```python
from build123d import *

# Parameters (mm, degrees)
SALIENTE_EXTRUIR2_DEPTH = 10
ESCALA1_SCALE           = 0.5


with BuildPart() as part:
    # Croquis1 → Saliente-Extruir2 (new body)
    with BuildSketch(Plane(origin=(0, 0, 0), x_dir=(1, 0, 0), z_dir=(0, 1, 0))):
        with BuildLine():
            Line((347.768463119, -7.519240019), (347.768463119, 12.480759981))
            Line((347.768463119, 12.480759981), (-82.231536881, 17.480759981))
            Line((-82.231536881, 17.480759981), (-89.231536881, 17.480759981))
            ThreePointArc((-89.231536881, 17.480759981), (-89.938643662, 17.187866762), (-90.231536881, 16.480759981))
            Line((-90.231536881, 16.480759981), (-90.231536881, 13.480759981))
            ThreePointArc((-90.231536881, 13.480759981), (-89.938643662, 12.7736532), (-89.231536881, 12.480759981))
            Line((-89.231536881, 12.480759981), (-82.231536881, 12.480759981))
            Line((-82.231536881, 12.480759981), (-82.231536881, -7.519240019))
            Line((-82.231536881, -7.519240019), (-89.231536881, -7.519240019))
            ThreePointArc((-89.231536881, -7.519240019), (-89.938643662, -7.812133238), (-90.231536881, -8.519240019))
            Line((-90.231536881, -8.519240019), (-90.231536881, -11.519240019))
            ThreePointArc((-90.231536881, -11.519240019), (-89.938643662, -12.2263468), (-89.231536881, -12.519240019))
            Line((-89.231536881, -12.519240019), (-82.231536881, -12.519240019))
            Line((-82.231536881, -12.519240019), (347.768463119, -7.519240019))
        make_face()
        Polygon((-35.970310827, -6.981318786), (-35.970310827, 11.942838748), (-59.970310827, 12.221908515), (-59.970310827, -7.260388554), align=None, mode=Mode.SUBTRACT)
        Polygon((-6.36676246, -6.637091479), (-6.36676246, 11.598611441), (-30.970310827, 11.884699213), (-30.970310827, -6.923179251), align=None, mode=Mode.SUBTRACT)
        Polygon((24.032508683, -6.283611582), (24.032508683, 11.245131544), (-1.36676246, 11.540471906), (-1.36676246, -6.578951945), align=None, mode=Mode.SUBTRACT)
        Polygon((54.471653082, -5.929668043), (54.471653082, 10.891188004), (29.032508683, 11.186992009), (29.032508683, -6.225472048), align=None, mode=Mode.SUBTRACT)
        Polygon((83.209124846, -5.595511395), (83.209124846, 10.557031356), (59.471653082, 10.83304847), (59.471653082, -5.871528508), align=None, mode=Mode.SUBTRACT)
        Polygon((112.395607474, -5.25613369), (112.395607474, 10.217653651), (88.209124846, 10.498891821), (88.209124846, -5.53737186), align=None, mode=Mode.SUBTRACT)
        Polygon((142.246515855, -4.909030104), (142.246515855, 9.870550065), (117.395607474, 10.159514116), (117.395607474, -5.197994155), align=None, mode=Mode.SUBTRACT)
        Polygon((171.437834583, -4.569596165), (171.437834583, 9.531116127), (147.246515855, 9.81241053), (147.246515855, -4.850890569), align=None, mode=Mode.SUBTRACT)
        Polygon((200.288401316, -4.234124459), (200.288401316, 9.19564442), (176.437834583, 9.472976592), (176.437834583, -4.51145663), align=None, mode=Mode.SUBTRACT)
        Polygon((229.28834427, -3.89691582), (229.28834427, 8.858435781), (205.288401316, 9.137504885), (205.288401316, -4.175984924), align=None, mode=Mode.SUBTRACT)
        Polygon((258.357613703, -3.558901059), (258.357613703, 8.52042102), (234.28834427, 8.800296246), (234.28834427, -3.838776285), align=None, mode=Mode.SUBTRACT)
        Polygon((287.325919365, -3.222060295), (287.325919365, 8.183580257), (263.357613703, 8.462281486), (263.357613703, -3.500761524), align=None, mode=Mode.SUBTRACT)
        Polygon((315.709556101, -2.892018008), (315.709556101, 7.853537969), (292.325919365, 8.125440722), (292.325919365, -3.163920761), align=None, mode=Mode.SUBTRACT)
        Polygon((342.768463119, -2.577379554), (342.768463119, 7.538899516), (320.709556101, 7.795398434), (320.709556101, -2.833878473), align=None, mode=Mode.SUBTRACT)
        Polygon((-64.970310827, -7.318528088), (-64.970310827, 12.28004805), (-72.387230354, 12.3662913), (-79.231536881, 6.910670608), (-79.231536881, -1.949150646), (-72.387230358, -7.404771339), align=None, mode=Mode.SUBTRACT)
    extrude(amount=SALIENTE_EXTRUIR2_DEPTH)


with BuildPart() as part_1:
    # Escala1: scaled about (123.080377325, 5, -2.480759981)
    add(part.part.scale(ESCALA1_SCALE).moved(Location((61.540188663, 2.5, -1.24037999))))


solid = part_1.part
```
Here's how the part is built. I have some questions about the finished solid (model axes, mm). Coordinates: 2 decimals unless noted, no trailing zeros. Order: outer loops, then holes, each group sorted by start corner. A loop starts at its lowest first (then second) coordinate and runs counter-clockwise, first axis right, second up.
1) Imagine slicing it at A-A on x = 36.5. List the corners of the cut face in (y, z) for me.
2) Will this pin go through, and if not, where does the flat tip stop? pin 1 (2.5 mm diameter, centred on y = 5, z = -0.5, fed in from -X).
3) I need wall thicknesses on line 1 (Z direction, x = 34, y = 7.15); line 2 (Z direction, x = 171, y = 6.45); line 3 (Z direction, x = 192, y = 2.85). Which ranges of each line are inside material? Lowest first, please.
4) Imagine slicing it at B-B on y = 4.6. State how many separate pieces and enclosed holes the cut face has, and give its area (3 significant figures).
Response values:
1. outline: (2.5, -9.79) - (7.5, -9.79) - (7.5, -7.29) - (2.5, -7.29) - close; (2.5, 2.33) - (7.5, 2.33) - (7.5, 4.83) - (2.5, 4.83) - close
2. pin 1: stops at x = 20.42
3. line 1: z = -9.82 to -7.32, 2.36 to 4.86
3. line 2: z = -8.23 to -5.73, 0.77 to 3.27
3. line 3: z = -7.99 to 3.02
4. separate pieces: 1
4. enclosed holes: 15
4. area: 1,400 mm2
